Autodesk Inventor part; units mm, degrees
ref_plane "YZ Plane" through (0, 0, 0) normal (1, 0, 0) x (0, 1, 0)
ref_plane "XZ Plane" through (0, 0, 0) normal (0, 1, 0) x (-1, 0, 0)
ref_plane "XY Plane" through (0, 0, 0) normal (0, 0, 1) x (1, 0, 0)
sketch "Sketch1" plane through (0, 0, 0) normal (0, 0, 1) x (1, 0, 0)
  circle A0 centre (37.4, -51.5) radius 1.75
  circle A1 centre (37.4, 51.5) radius 1.75
  circle A2 centre (-37.4, -51.5) radius 1.75
  circle A3 centre (-37.4, 51.5) radius 1.75
  line L0 (-32.4, 44.5) -> (-32.4, -44.5)
  line L1 (-34.4, -46.5) -> (-40.4, -46.5)
  line L2 (-42.4, -48.5) -> (-42.4, -54.5)
  line L3 (-40.4, -56.5) -> (40.4, -56.5)
  line L4 (42.4, -54.5) -> (42.4, -48.5)
  line L5 (40.4, -46.5) -> (34.4, -46.5)
  line L6 (32.4, -44.5) -> (32.4, 44.5)
  line L7 (34.4, 46.5) -> (40.4, 46.5)
  line L8 (42.4, 48.5) -> (42.4, 54.5)
  line L9 (40.4, 56.5) -> (-40.4, 56.5)
  line L10 (-42.4, 54.5) -> (-42.4, 48.5)
  line L11 (-40.4, 46.5) -> (-34.4, 46.5)
  line L12 (30.4, -54.5) -> (-30.4, -54.5)
  line L13 (-30.4, -54.5) -> (-30.4, 54.5)
  line L14 (-30.4, 54.5) -> (30.4, 54.5)
  line L15 (30.4, 54.5) -> (30.4, -54.5)
  arc A4 (40.4, -56.5) -> (42.4, -54.5) centre (40.4, -54.5) ccw
  arc A5 (42.4, -48.5) -> (40.4, -46.5) centre (40.4, -48.5) ccw
  arc A6 (32.4, -44.5) -> (34.4, -46.5) centre (34.4, -44.5) ccw
  arc A7 (34.4, 46.5) -> (32.4, 44.5) centre (34.4, 44.5) ccw
  arc A8 (40.4, 46.5) -> (42.4, 48.5) centre (40.4, 48.5) ccw
  arc A9 (42.4, 54.5) -> (40.4, 56.5) centre (40.4, 54.5) ccw
  arc A10 (-40.4, 56.5) -> (-42.4, 54.5) centre (-40.4, 54.5) ccw
  arc A11 (-42.4, 48.5) -> (-40.4, 46.5) centre (-40.4, 48.5) ccw
  arc A12 (-32.4, 44.5) -> (-34.4, 46.5) centre (-34.4, 44.5) ccw
  arc A13 (-34.4, -46.5) -> (-32.4, -44.5) centre (-34.4, -44.5) ccw
  arc A14 (-40.4, -46.5) -> (-42.4, -48.5) centre (-40.4, -48.5) ccw
  arc A15 (-42.4, -54.5) -> (-40.4, -56.5) centre (-40.4, -54.5) ccw
  point P0 (0, 0)
extrude "Extrusion1" add sketch "Sketch1" along normal blind 3 contours A12 L11 A11 L10 A10 L9 A9 L8 A8 L7 A7 L6 A6 L5 A5 L4 A4 L3 A15 L2 A14 L1 A13 L0 | L12 L13 L14 L15
sketch "Sketch2" plane through (0, 0, 0) normal (0, 0, -1) x (-1, 0, 0)
  circle A0 centre (26.3, -50.4) radius 1.5
  circle A1 centre (-26.3, -50.4) radius 1.5
  circle A2 centre (-26.3, 50.4) radius 1.5
  circle A3 centre (26.3, 50.4) radius 1.5
  circle A4 centre (26.3, -50.4) radius 1.25
  circle A5 centre (-26.3, -50.4) radius 1.25
  circle A6 centre (-26.3, 50.4) radius 1.25
  circle A7 centre (26.3, 50.4) radius 1.25
  circle A8 centre (-26.3, -50.4) radius 2
  circle A9 centre (26.3, -50.4) radius 2
  circle A10 centre (26.3, 50.4) radius 2
  circle A11 centre (-26.3, 50.4) radius 2
  point P0 (0, 0)
  dimension "d2" = 2.5
  dimension "d3" = 4
extrude "Extrusion2" add sketch "Sketch2" along normal blind 2.1 contours A0 | A1 | A2 | A3 | A4 | A5 | A6 | A7 | A8 | A9 | A10 | A11
fillet "Fillet1" radius 1.5 4 edges at (28.3, -50.4, 0) (-24.3, -50.4, 0) (-24.3, 50.4, 0) (28.3, 50.4, 0)
sketch "Sketch3" plane through (-26.3, -50.4, 0) normal (0, 0, -1) x (-1, 0, 0)
  circle A0 centre (0, 0) radius 2
  circle A1 centre (0, 0) radius 1.25
  circle A2 centre (-52.6, 0) radius 1.25
  circle A3 centre (-52.6, 100.8) radius 1.25
  circle A4 centre (0, 100.8) radius 1.25
  point P0 (-26.3, 50.4)
extrude "Extrusion3" add sketch "Sketch3" along normal blind 5 contours A1 | A2 | A3 | A4
properties part number "CAJA_P2"
Here's how the part is built. I have some questions about the finished solid (model axes, mm). A direction names the side the tool comes from. Coordinates: 2 decimals unless noted, no trailing zeros. Write each loop counter-clockwise with the first axis right and the second up, starting at its lowest first coordinate (ties: lowest second). Pieces come first, ordered by that corner, then holes.
Item 1: I want a section at C-C on y = -34.5. Write out the boundary of the cut face in (x, z), and give its area (3 significant figures).
Item 2: If we mould it in two halves opening along X, with no side actions, what happens to faces 6 (the cylindrical face through (-24.7, 51.6, -1.8)), 7 (the flat face through (37, 46.5, 1)), 8 (the flat face through (-42.4, 52, 1))? For each: +X half, -X half, draft (parallel to the pull), parting line (faces both ways), or undercut.
Item 3: On a 3-axis mill with a long thin cutter (end or side, diameter ignored), from which of +Z, -Z, +X, -X, +Y, -Y can I reach the whole of each face in a straight line? I mean faces 1 (the flat face through (-1, -56.5, 1)), 2 (the cylindrical face through (-36.59, 53.05, 1.48)), 3 (the flat face through (-37, 46.5, 1)), 4 (the cylindrical face through (-26.03, 51.62, -3.53)), 5 (the flat face through (37, -46.5, 1)). Say none if no direction works.
Item 4: I want a section at B-B on x = -26.3. Write out the boundary of the cut face in (y, z), and give its area (3 significant figures).
Item 5: Will these pins go through, and if not, where does the flat tip stop? pin 1 (4.5 mm diameter, centred on x = -37.4, y = -51.5, fed in from -Z); pin 2 (0.9 mm diameter, centred on y = -14.5, z = 1.5, fed in from +X); pin 3 (3.5 mm diameter, centred on y = 5.5, z = 1.5, fed in from -X); pin 4 (1 mm diameter, centred on x = -8.5, z = -1, fed in from -Y).
Item 6: I want a section at A-A on x = 37.4. Write out the boundary of the cut face in (y, z).
Item 7: If I drill on line 1 (Y direction, x = -37.4, z = 1.95); line 2 (Y direction, x = -36, z = 2.75); line 3 (Z direction, x = 31, y = -13.5), over which ranges is the centre line in solid material (lowest first)?
Item 8: I want a section at D-D on x = -1. Write out the boundary of the cut face in (y, z), and give its area (3 significant figures).
Findings below:
1. outline: (-32.4, 0) - (32.4, 0) - (32.4, 3) - (-32.4, 3) - close
1. area: 194 mm2
2. face 6: undercut
2. face 7: draft
2. face 8: -X half
3. face 1: +Z, -Z, +X, -X, -Y
3. face 2: +Z, -Z
3. face 3: +Z, -Z, -X
3. face 4: -Z
3. face 5: +Z, -Z, +X
4. outline: (-56.5, 0) - (-53.9, 0) arc R1.5 cw to (-52.4, -1.5) - (-52.4, -2.1) - (-51.65, -2.1) - (-51.65, -5) - (-49.15, -5) - (-49.15, -2.1) - (-48.4, -2.1) - (-48.4, -1.5) arc R1.5 cw to (-46.9, 0) - (46.9, 0) arc R1.5 cw to (48.4, -1.5) - (48.4, -2.1) - (49.15, -2.1) - (49.15, -5) - (51.65, -5) - (51.65, -2.1) - (52.4, -2.1) - (52.4, -1.5) arc R1.5 cw to (53.9, 0) - (56.5, 0) - (56.5, 3) - (-56.5, 3) - close
4. area: 372 mm2
5. pin 1: stops at z = 0
5. pin 2: stops at x = 32.4
5. pin 3: stops at x = -32.4
5. pin 4: passes through
6. outline: (-56.5, 0) - (-53.25, 0) - (-53.25, 3) - (-56.5, 3) - close; (-49.75, 0) - (-46.5, 0) - (-46.5, 3) - (-49.75, 3) - close; (46.5, 0) - (49.75, 0) - (49.75, 3) - (46.5, 3) - close; (53.25, 0) - (56.5, 0) - (56.5, 3) - (53.25, 3) - close
7. line 1: y = -56.5 to -53.25, -49.75 to -46.5, 46.5 to 49.75, 53.25 to 56.5
7. line 2: y = -56.5 to -52.55, -50.45 to -46.5, 46.5 to 50.45, 52.55 to 56.5
7. line 3: z = 0 to 3
8. outline: (-56.5, 0) - (56.5, 0) - (56.5, 3) - (-56.5, 3) - close
8. area: 339 mm2
